Design review of the part built by this model. Coordinates are the model's own, in mm. Face numbers are marked on the shaded views. Round coordinates to 2 decimals unless told otherwise and drop trailing zeros. Write each loop counter-clockwise with the first axis right and the second up, starting at its lowest first coordinate (ties: lowest second). Pieces come first, ordered by that corner, then holes. Notation, with made-up numbers: M 37,59.25 L 46,59.25 A27 cw 46,87.25 Z; hole C 24,31 d2. An arc over 180 degrees is marked long. Use CSV: the item, a comma, the result in double quotes.
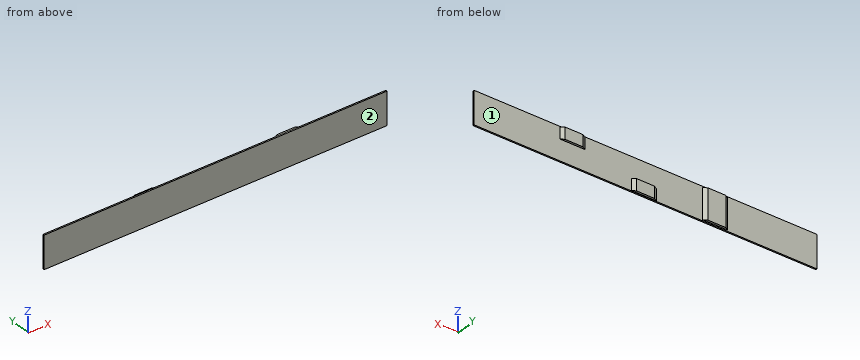
from build123d import *

# Parameters (mm, degrees)
SKETCH1_W                = 2400
SKETCH1_H                = 225
BOSS_EXTRUDE1_DEPTH      = 10
BOSS_EXTRUDE2_START      = 30
BOSS_EXTRUDE2_DEPTH      = 80
BOSS_EXTRUDE3_START      = -30
BOSS_EXTRUDE3_DEPTH      = 80
BOSS_EXTRUDE4_DEPTH      = 105
BOSS_EXTRUDE4_DEPTH_BACK = 105


with BuildPart() as part:
    # Sketch1 → Boss-Extrude1 (new body)
    with BuildSketch(Plane(origin=(0, 0, 0), x_dir=(1, 0, 0), z_dir=(0, 1, 0))):
        Rectangle(SKETCH1_W, SKETCH1_H)
    extrude(amount=BOSS_EXTRUDE1_DEPTH)

    # Sketch2 → Boss-Extrude2 (add)
    with BuildSketch(Plane.XY.offset(BOSS_EXTRUDE2_START)):
        Polygon((425, 10), (600, 10), (575, 25), (450, 25), align=None)
    extrude(amount=BOSS_EXTRUDE2_DEPTH)

    # Sketch4 → Boss-Extrude3 (add)
    with BuildSketch(Plane.XY.offset(BOSS_EXTRUDE3_START)):
        Polygon((100, 10), (75, 25), (-50, 25), (-75, 10), align=None)
    extrude(amount=-BOSS_EXTRUDE3_DEPTH)

    # Sketch5 → Boss-Extrude4 (add, two sides: drawn at the far end of the back side and taken through both)
    with BuildSketch(Plane.XY.offset(-BOSS_EXTRUDE4_DEPTH_BACK)):
        Polygon((-575, 10), (-400, 10), (-425, 25), (-550, 25), align=None)
    extrude(amount=BOSS_EXTRUDE4_DEPTH + BOSS_EXTRUDE4_DEPTH_BACK)


solid = part.part
1) Add section A-A on z = -57.5. Write out the cut boundary in (x, y), then the cut area to 3 significant figures.
Answers:
outline,"M -1200,0 L 1200,0 L 1200,10 L 100,10 L 75,25 L -50,25 L -75,10 L -400,10 L -425,25 L -550,25 L -575,10 L -1200,10 Z"
area,"28,500 mm²"
2) Add section C-C on x = 0.5. Write out the cut boundary in (y, z).
Answers:
outline,"M 0,-112.5 L 10,-112.5 L 10,-110 L 25,-110 L 25,-30 L 10,-30 L 10,112.5 L 0,112.5 Z"
3) The part is to be moulded in two halves that separate along X. For the marked faces 1 and 2, say which applies: released by +X, released by -X, zero draft, split by the parting line, or undercut.
Answers:
face 1,"undercut"
face 2,"zero draft"
4) For pin 1 Ø12 at (x, z) = (-13.5, -52) entering from -Y; pin 2 Ø7.5 at (x, y) = (52.5, 20) entering from +Z; pin 3 Ø1.5 at (x, z) = (30, 49) entering from +Y; pin 4 Ø12 at (x, y) = (503.5, 18.5) entering from -Z, all flat-tipped, find the tip position at first contact; note any pin that passes through.
Answers:
pin 1,"y = 0"
pin 2,"z = -30"
pin 3,"y = 10"
pin 4,"z = 30"
5) Add section D-D on x = -843.5. Write out the cut boundary in (y, z), then the cut area to 3 significant figures.
Answers:
outline,"M 0,-112.5 L 10,-112.5 L 10,112.5 L 0,112.5 Z"
area,"2,250 mm²"
6) Wall thickness on line 1 along Y through (x, z) = (-339, -81); line 2 along X through (y, z) = (20.5, 47); line 3 along Z through (x, y) = (-510.5, 16): over which ranges is each line inside the solid? List them lowest first. Write a range as [from, to].
Answers:
line 1,"[0, 10]"
line 2,"[-557.5, -417.5], [442.5, 582.5]"
line 3,"[-105, 105]"
7) Add section B-B on y = 16.5. Write out the cut boundary in (x, z), then the cut area to 3 significant figures.
Answers:
outline,"M -564.17,-105 L -410.83,-105 L -410.83,105 L -564.17,105 Z; M -64.17,-110 L 89.17,-110 L 89.17,-30 L -64.17,-30 Z; M 435.83,30 L 589.17,30 L 589.17,110 L 435.83,110 Z"
area,"56,700 mm²"
